Can you work these out from the model? Positions are in its coordinate system, mm. A direction names the side the tool comes from. Round coordinates to 2 decimals unless told otherwise and drop trailing zeros. Loops run counter-clockwise (first coordinate to the right, second up) from the corner with the lowest first, then second, coordinate; pieces in that order, holes last.
(1) Will this pin go through, and if not, where does the flat tip stop? pin 1 Ø1 at (x, y) = (10, 51) entering from -Z.
(2) I want a section at B-B on y = 38. Write out the boundary of the cut face in (x, z).
(3) I want a section at C-C on z = 154. Write out the boundary of the cut face in (x, y).
(4) Which directions (+Z, -Z, +X, -X, +Y, -Y) give clear straight access to the entire face, cutting with the end or side of a thin tool? Please do faces 5 (the face through (17.255, 41.562, 219.306)), 6 (the face through (17, 0, 129)), 7 (the face through (17.255, 57.594, 220.667)).
(5) I want a section at D-D on y = 16.5. Write out the boundary of the cut face in (x, z).
(6) If I drill on line 1 along X through (y, z) = (41, 190.5); line 2 along Z through (x, y) = (29, 35.5); line 3 along Z through (x, y) = (31.5, 13.5), over which ranges is the centre line in solid material (lowest first)?
(7) I want a section at A-A on x = 3.5. Write out the boundary of the cut face in (y, z), plus the area to 3 significant figures.
(8) Thinking about a two-plate mould opening in X: for faces 1 (the face through (17.255, 33.134, 165.049)), 2 (the face through (17, 30, 0)), 3 (the face through (-15, 30, 125)), 4 (the face through (17.26, 30.56, 210.2)), which applies, released by +X, released by -X, zero draft, split by the parting line, or undercut?
from build123d import *

# Parameters (mm, degrees)
F1_DEPTH = 35
F2_W     = 15
F2_H     = 254
F3_DEPTH = 60


with BuildPart() as f1:
    # F0 (on Right) → F1 (new body)
    with BuildSketch(Plane.YZ):
        with BuildLine():
            Line((0, 254), (0, 0))
            Line((0, 0), (60, 0))
            Line((60, 0), (60, 133.360773))
            ThreePointArc((60, 133.360773), (32.79815, 165.535249), (12.434966, 202.419911))
            ThreePointArc((12.434966, 202.419911), (10.913963, 203.546609), (11.548571, 205.329913))
            Line((11.548571, 205.329913), (25.72096, 208.454538))
            ThreePointArc((25.72096, 208.454538), (30.629217, 210.234525), (34.909535, 213.22421))
            Line((34.909535, 213.22421), (48.403102, 225.559899))
            ThreePointArc((48.403102, 225.559899), (49.665358, 225.965052), (50.795926, 225.272772))
            Line((50.795926, 225.272772), (52.84946, 222.214688))
            ThreePointArc((52.84946, 222.214688), (53.089616, 221.021687), (52.415852, 220.008292))
            Line((52.415852, 220.008292), (50, 218.386023))
            Line((50, 218.386023), (52, 218.386023))
            ThreePointArc((52, 218.386023), (57.656854, 220.729169), (60, 226.386023))
            Line((60, 226.386023), (60, 254))
            Line((60, 254), (0, 254))
        make_face()
    extrude(amount=F1_DEPTH)

    # F2 (on face) → F3 (join)
    with BuildSketch(Plane.XZ):
        with Locations((-7.5, 127)):
            Rectangle(F2_W, F2_H)
        with Locations((42.5, 127)):
            Rectangle(F2_W, F2_H)
    extrude(amount=-F3_DEPTH)


solid = f1.part
Filled sheet:
1. pin 1: stops at z = 0
2. outline: (-15, 0) - (50, 0) - (50, 254) - (-15, 254) - close; hole (0, 158.31) - (35, 158.31) - (35, 216.05) - (0, 216.05) - close
3. outline: (-15, 0) - (50, 0) - (50, 60) - (35, 60) - (35, 41.33) - (0, 41.33) - (0, 60) - (-15, 60) - close
4. face 5: none
4. face 6: +Z, -Z, +X, -X, -Y
4. face 7: +Y
5. outline: (-15, 0) - (50, 0) - (50, 254) - (-15, 254) - close; hole (0, 193.52) - (35, 193.52) - (35, 206.42) - (0, 206.42) - close
6. line 1: x = -15 to 0, 35 to 50
6. line 2: z = 0 to 161.7, 213.76 to 254
6. line 3: z = 0 to 199.98, 205.76 to 254
7. outline: (0, 0) - (60, 0) - (60, 133.36) arc R213.77 cw to (12.43, 202.42) arc R1.59 cw to (11.55, 205.33) - (25.72, 208.45) arc R20 ccw to (34.91, 213.22) - (48.4, 225.56) arc R1.59 cw to (50.8, 225.27) - (52.85, 222.21) arc R1.59 cw to (52.42, 220.01) - (50, 218.39) - (52, 218.39) arc R8 ccw to (60, 226.39) - (60, 254) - (0, 254) - close
7. area: 12,800 mm2
8. face 1: undercut
8. face 2: zero draft
8. face 3: released by -X
8. face 4: undercut
